Could you check a few things on this model? Use its own coordinates, in mm. A direction names the side the tool comes from. Coordinates: 2 decimals unless noted, no trailing zeros. Loops run counter-clockwise (first coordinate to the right, second up) from the corner with the lowest first, then second, coordinate; pieces in that order, holes last. Notation, with made-up numbers: (19.5, 61) -> (48.5, 61) arc R25 ccw to (48.5, 100) -> close; hole circle Ø10 at (40, 85.25). An arc over 180 degrees is marked (long way). One line per question, with ' | ' between items.
from build123d import *

# Parameters (mm, degrees)
SKETCH2_W           = 111.125
SKETCH2_H           = 55.88
SKETCH2_R           = 3.81
BOSS_EXTRUDE1_DEPTH = 25.4
SKETCH4_R           = 15.24
CUT_EXTRUDE2_DEPTH  = 17.78
CUT_EXTRUDE3_DEPTH  = 17.78
SKETCH6_R           = 6.35
CUT_EXTRUDE4_DEPTH  = 20.32
SKETCH7_R           = 14.3002
CUT_EXTRUDE5_DEPTH  = 2.54
SKETCH8_R           = 6.35
CUT_EXTRUDE6_DEPTH  = 23.86
SKETCH9_R           = 11.43
SKETCH9_R_2         = 6.35
CUT_EXTRUDE7_DEPTH  = 17.78
SKETCH10_R          = 2.5
CUT_EXTRUDE8_DEPTH  = 26.4


with BuildPart() as part:
    # Sketch2 → Boss-Extrude1 (new body)
    with BuildSketch(Plane.XY):
        with Locations((55.5625, 27.94)):
            Rectangle(SKETCH2_W, SKETCH2_H)
        with Locations((12.7, 46.355)):
            Circle(SKETCH2_R, mode=Mode.SUBTRACT)
        with BuildLine():
            Line((70.988225187, 41.8465), (64.638225187, 41.8465))
            ThreePointArc((64.638225187, 41.8465), (63.050725187, 43.434), (64.638225187, 45.0215))
            Line((64.638225187, 45.0215), (70.988225187, 45.0215))
            ThreePointArc((70.988225187, 45.0215), (72.575725187, 43.434), (70.988225187, 41.8465))
        make_face(mode=Mode.SUBTRACT)
        with BuildLine():
            Line((101.976225187, 41.8465), (95.626225187, 41.8465))
            ThreePointArc((95.626225187, 41.8465), (94.038725187, 43.434), (95.626225187, 45.0215))
            Line((95.626225187, 45.0215), (101.976225187, 45.0215))
            ThreePointArc((101.976225187, 45.0215), (103.563725187, 43.434), (101.976225187, 41.8465))
        make_face(mode=Mode.SUBTRACT)
        with BuildLine():
            Line((101.976225187, 10.8585), (95.626225187, 10.8585))
            ThreePointArc((95.626225187, 10.8585), (94.038725187, 12.446), (95.626225187, 14.0335))
            Line((95.626225187, 14.0335), (101.976225187, 14.0335))
            ThreePointArc((101.976225187, 14.0335), (103.563725187, 12.446), (101.976225187, 10.8585))
        make_face(mode=Mode.SUBTRACT)
        with BuildLine():
            Line((70.988225187, 10.8585), (64.638225187, 10.8585))
            ThreePointArc((64.638225187, 10.8585), (63.050725187, 12.446), (64.638225187, 14.0335))
            Line((64.638225187, 14.0335), (70.988225187, 14.0335))
            ThreePointArc((70.988225187, 14.0335), (72.575725187, 12.446), (70.988225187, 10.8585))
        make_face(mode=Mode.SUBTRACT)
    extrude(amount=BOSS_EXTRUDE1_DEPTH)

    # Sketch4 → Cut-Extrude2 (cut)
    with BuildSketch(Plane(origin=(0, 0, 0), x_dir=(-1, 0, 0), z_dir=(0, 0, -1))):
        with Locations((-12.7, 46.355)):
            Circle(SKETCH4_R)
    extrude(amount=-CUT_EXTRUDE2_DEPTH, mode=Mode.SUBTRACT)

    # Sketch5 → Cut-Extrude3 (cut)
    with BuildSketch(Plane(origin=(0, 0, 0), x_dir=(-1, 0, 0), z_dir=(0, 0, -1))):
        with BuildLine():
            Line((0, 54.779226968), (0, 55.88))
            Line((0, 55.88), (-0.803278813, 55.88))
            ThreePointArc((-0.803278813, 55.88), (-0.389329888, 55.33859624), (0, 54.779226968))
        make_face()
    extrude(amount=-CUT_EXTRUDE3_DEPTH, mode=Mode.SUBTRACT)

    # Sketch6 → Cut-Extrude4 (cut)
    with BuildSketch(Plane(origin=(0, 0, 0), x_dir=(-1, 0, 0), z_dir=(0, 0, -1))):
        with Locations((-98.801225187, 43.434)):
            Circle(SKETCH6_R)
        with Locations((-98.801225187, 12.446)):
            Circle(SKETCH6_R)
        with Locations((-67.813225187, 43.434)):
            Circle(SKETCH6_R)
        with Locations((-67.813225187, 12.446)):
            Circle(SKETCH6_R)
    extrude(amount=-CUT_EXTRUDE4_DEPTH, mode=Mode.SUBTRACT)

    # Sketch7 → Cut-Extrude5 (cut)
    with BuildSketch(Plane.XY.offset(25.4)):
        with Locations((83.307225187, 27.94)):
            Circle(SKETCH7_R)
    extrude(amount=-CUT_EXTRUDE5_DEPTH, mode=Mode.SUBTRACT)

    # Sketch8 → Cut-Extrude6 (cut, through all)
    with BuildSketch(Plane.XY.offset(22.86)):
        with Locations((83.307225187, 27.94)):
            Circle(SKETCH8_R)
    extrude(amount=-CUT_EXTRUDE6_DEPTH, mode=Mode.SUBTRACT)

    # Sketch9 → Cut-Extrude7 (cut)
    with BuildSketch(Plane(origin=(0, 0, 0), x_dir=(-1, 0, 0), z_dir=(0, 0, -1))):
        with Locations((-83.307225187, 27.94)):
            Circle(SKETCH9_R)
        with Locations((-83.307225187, 27.94)):
            Circle(SKETCH9_R_2, mode=Mode.SUBTRACT)
        with BuildLine():
            Line((-74.135687658, 42.843264609), (-86.765332472, 38.834328525))
            ThreePointArc((-86.765332472, 38.834328525), (-76.557457275, 37.164181976), (-71.877225187, 27.94))
            ThreePointArc((-71.877225187, 27.94), (-74.448057171, 20.717809053), (-81.004091691, 16.744443913))
            Line((-81.004091691, 16.744443913), (-9.629155339, 31.427591884))
            ThreePointArc((-9.629155339, 31.427591884), (-25.698234103, 38.398649693), (-24.596721187, 55.88))
            Line((-24.596721187, 55.88), (-33.065105822, 55.88))
            Line((-33.065105822, 55.88), (-62.307510769, 46.597796572))
            ThreePointArc((-62.307510769, 46.597796572), (-61.677926231, 45.071255852), (-61.463225187, 43.434))
            ThreePointArc((-61.463225187, 43.434), (-67.517536745, 37.090888118), (-74.135687658, 42.843264609))
        make_face()
    extrude(amount=-CUT_EXTRUDE7_DEPTH, mode=Mode.SUBTRACT)

    # Sketch10 → Cut-Extrude8 (cut, through all)
    with BuildSketch(Plane.XY.offset(25.4)):
        with Locations((5.08, 5.08)):
            Circle(SKETCH10_R)
        with Locations((20.32, 5.08)):
            Circle(SKETCH10_R)
        with Locations((20.32, 22.86)):
            Circle(SKETCH10_R)
        with Locations((5.08, 22.86)):
            Circle(SKETCH10_R)
    extrude(amount=-CUT_EXTRUDE8_DEPTH, mode=Mode.SUBTRACT)


solid = part.part
1) If we section it at A-A on y = 5.08: Please give me the cut outline in (x, z) (3 decimals), and give its area (3 significant figures).
Data:
outline: (0, 0) -> (2.58, 0) -> (2.58, 25.4) -> (0, 25.4) -> close; (7.58, 0) -> (17.82, 0) -> (17.82, 25.4) -> (7.58, 25.4) -> close; (22.82, 0) -> (111.125, 0) -> (111.125, 25.4) -> (22.82, 25.4) -> close | area: 2,570 mm²
2) If we section it at D-D on z = 15: Please give me the cut outline in (x, y) (3 decimals).
Data:
outline: (0, 0) -> (111.125, 0) -> (111.125, 55.88) -> (33.065, 55.88) -> (62.308, 46.598) arc R6.35 cw to (74.136, 42.843) -> (86.765, 38.834) arc R11.43 cw to (81.004, 16.744) -> (9.629, 31.428) arc R15.24 cw to (0, 37.931) -> close; hole circle Ø5 at (5.08, 5.08); hole circle Ø5 at (5.08, 22.86); hole circle Ø5 at (20.32, 5.08); hole circle Ø5 at (20.32, 22.86); hole circle Ø12.7 at (67.813, 12.446); hole circle Ø12.7 at (98.801, 12.446); hole circle Ø12.7 at (98.801, 43.434)
3) We'd pull the mould along X, two halves only. Please class faces 1 (the face through (55, 16, 0)), 2 (the face through (111.125, 28, 13)), 3 (the face through (17.822, 22.97, 12.878)): pulls with the +X half, pulls with the -X half, needs draft (parallel to the pull), parting line crosses it, or undercut.
Data:
face 1: needs draft | face 2: pulls with the +X half | face 3: undercut
4) If we section it at B-B on x = 20.32: Please give me the cut outline in (y, z).
Data:
outline: (0, 0) -> (2.58, 0) -> (2.58, 25.4) -> (0, 25.4) -> close; (7.58, 0) -> (20.36, 0) -> (20.36, 25.4) -> (7.58, 25.4) -> close; (25.36, 0) -> (29.23, 0) -> (29.23, 17.78) -> (55.88, 17.78) -> (55.88, 25.4) -> (25.36, 25.4) -> close
5) On a 3-axis mill with a long thin cutter (end or side, diameter ignored), from which of +Z, -Z, +X, -X, +Y, -Y can I reach the whole of each face in a straight line? I mean faces 4 (the face through (86, 22, 22.86)), 5 (the face through (68.64, 49.73, 10.02)), 6 (the face through (68, 41.846, 23)), 7 (the face through (55, 28, 25.4)). Say none if no direction works.
Data:
face 4: +Z | face 5: -Z | face 6: +Z, -Z | face 7: +Z, +X, -X, +Y, -Y
6) I'm going to push flat-ended pins straight in: pin 1 Ø4 at (x, y) = (5.08, 22.86) entering from +Z; pin 2 Ø1.5 at (x, y) = (61.5, 42) entering from -Z; pin 3 Ø3 at (y, z) = (43.5, 3.5) entering from -X. Where does each tip first touch, or does it pass through?
Data:
pin 1: through | pin 2: z = 17.78 | pin 3: x = 73.97
7) If we section it at C-C on y = 22.86: Please give me the cut outline in (x, z) (3 decimals), and give its area (3 significant figures).
Data:
outline: (0, 0) -> (2.58, 0) -> (2.58, 25.4) -> (0, 25.4) -> close; (7.58, 0) -> (17.82, 0) -> (17.82, 25.4) -> (7.58, 25.4) -> close; (22.82, 0) -> (51.276, 0) -> (51.276, 17.78) -> (79.497, 17.78) -> (79.497, 22.86) -> (69.94, 22.86) -> (69.94, 25.4) -> (22.82, 25.4) -> close; (87.117, 17.78) -> (93.546, 17.78) -> (93.546, 0) -> (111.125, 0) -> (111.125, 25.4) -> (96.675, 25.4) -> (96.675, 22.86) -> (87.117, 22.86) -> close | area: 1,710 mm²
8) I need wall thicknesses on line 1 along Y through (x, z) = (20.32, 19.75); line 2 along X through (y, z) = (12, 13.75) (3 decimals); line 3 along X through (y, z) = (43, 8.5) (3 decimals). Which ranges of each line are inside material? Lowest first, please. Write a range as from..to.
Data:
line 1: 0..2.58, 7.58..20.36, 25.36..55.88 | line 2: 0..61.479, 74.148..92.467, 105.136..111.125 | line 3: 74.148..92.466, 105.136..111.125
